Verification items for this drawing (mm, ordinates from the low corner). A direction names the side the tool comes from. Coordinates: 2 decimals unless noted, no trailing zeros. Order: outer loops, then holes, each group sorted by start corner. A loop starts at its lowest first (then second) coordinate and runs counter-clockwise, first axis right, second up.
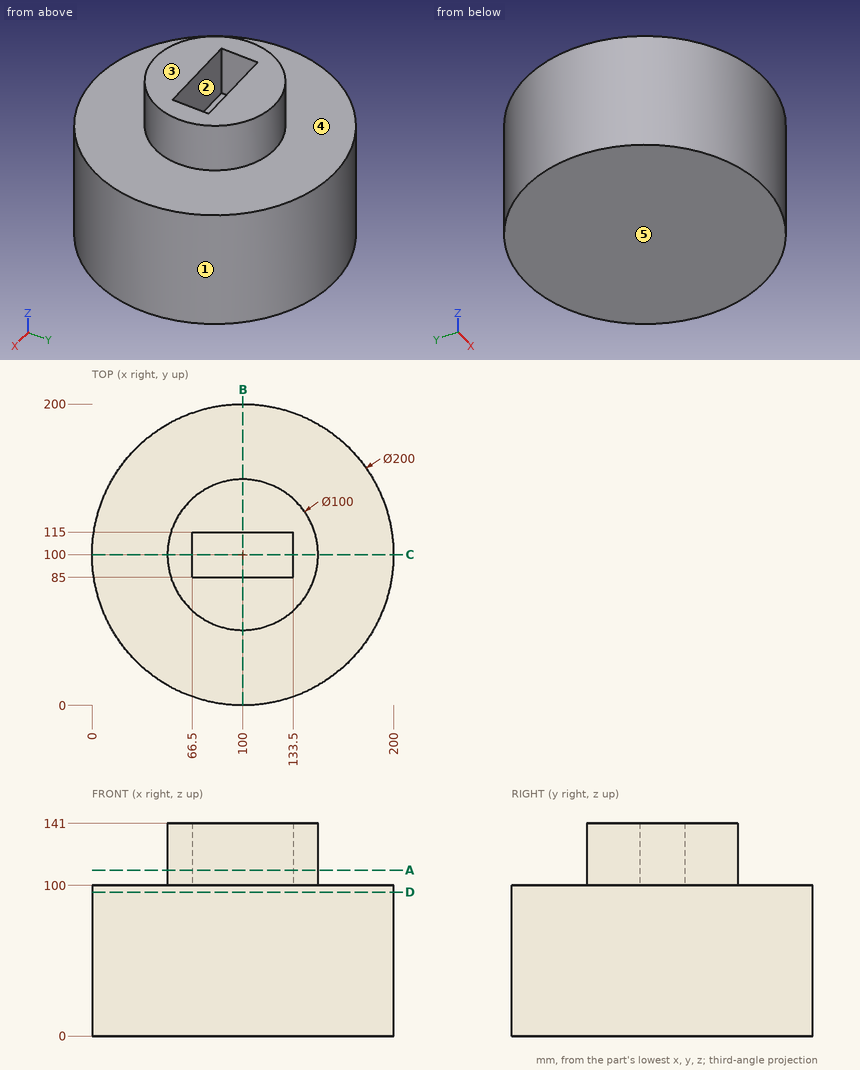
(1) Tool access check on the marked faces 4 and 5. Record the directions out of +Z, -Z, +X, -X, +Y, -Y that give a thin tool (end or side, any length) a straight path to the whole face; none if there is none.
Filled in:
face 4: +Z
face 5: -Z, +X, -X, +Y, -Y
(2) Cross-section at D-D (z = 95.5). Enter the section's corners in (x, y), and give its area (3 significant figures).
Filled in:
outline: circle Ø200 at (100, 100)
area: 31,400 mm2
(3) Thickness scan on probe 1 along Z at (x, y) = (165.5, 42.5); probe 2 along Y at (x, z) = (67, 105); probe 3 along Y at (x, z) = (77.5, 118). Record the ranges inside material, lowest first.
Filled in:
probe 1: z = 0 to 100
probe 2: y = 62.44 to 85, 115 to 137.56
probe 3: y = 55.35 to 85, 115 to 144.65
(4) Cross-section at B-B (x = 100). Enter the section's corners in (y, z), and give its area (3 significant figures).
Filled in:
outline: (0, 0) - (200, 0) - (200, 100) - (150, 100) - (150, 141) - (115, 141) - (115, 100) - (85, 100) - (85, 141) - (50, 141) - (50, 100) - (0, 100) - close
area: 22,900 mm2
(5) Go/stop test with flat-tipped pins: P1, Ø1, axis at y = 75.5, z = 17.5, coming from the -X side; P2, Ø5, axis at y = 84.5, z = 42.5, coming from the +X side; P3, Ø5, axis at x = 136.5, y = 159.5, coming from the -Z side; P4, Ø15, axis at y = 93.5, z = 120.5, coming from the -X side. Record where each tip stops, or that it passes through.
Filled in:
P1: stops at x = 2.92
P2: stops at x = 199.15
P3: stops at z = 0
P4: stops at x = 50
(6) Release check for a two-part mould opening along X. For the marked faces 1, 2 and 3 record: +X half, -X half, draft (parallel to the pull), parting line (faces both ways), or undercut.
Filled in:
face 1: parting line
face 2: undercut
face 3: draft
(7) Cross-section at C-C (y = 100). Enter the section's corners in (x, z), and give its area (3 significant figures).
Filled in:
outline: (0, 0) - (200, 0) - (200, 100) - (150, 100) - (150, 141) - (133.5, 141) - (133.5, 100) - (66.5, 100) - (66.5, 141) - (50, 141) - (50, 100) - (0, 100) - close
area: 21,400 mm2
(8) Cross-section at A-A (z = 110). Enter the section's corners in (x, y), and give its area (3 significant figures).
Filled in:
outline: circle Ø100 at (100, 100); hole (66.5, 85) - (133.5, 85) - (133.5, 115) - (66.5, 115) - close
area: 5,840 mm2
